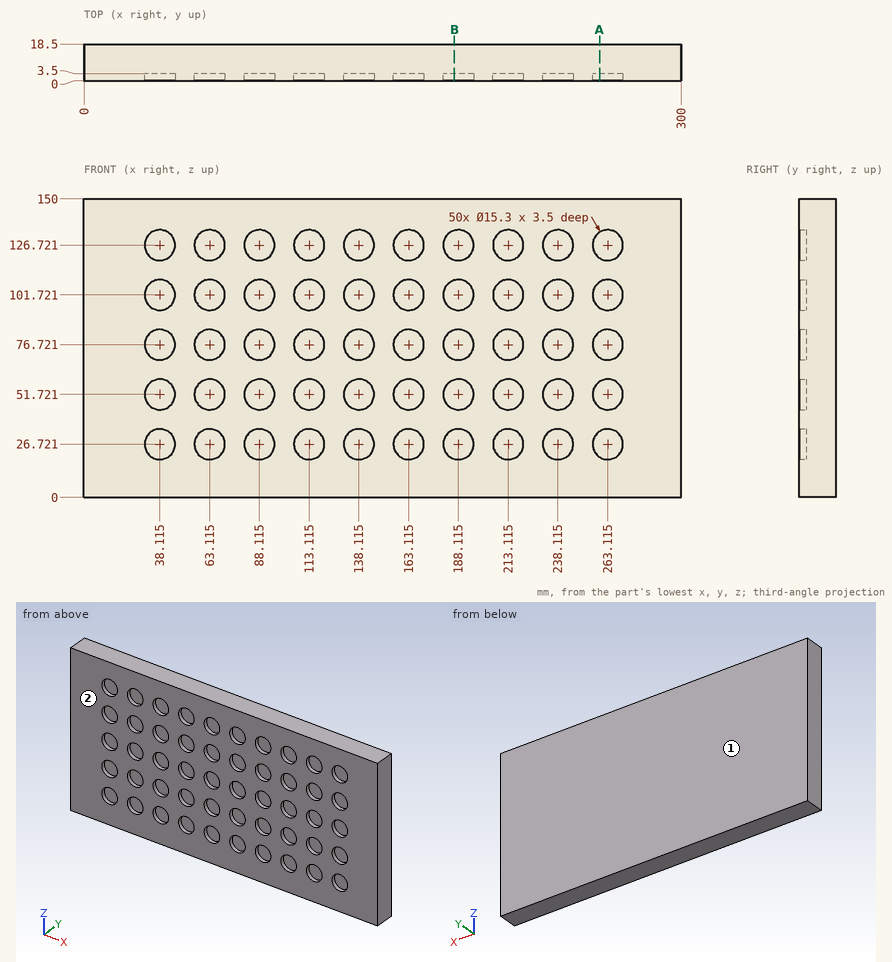
Can you work these out from the drawing? Everything is in mm from the part's minimum corner. Round coordinates to 2 decimals unless told otherwise and drop trailing zeros. Order: outer loops, then holes, each group sorted by start corner. A loop starts at its lowest first (then second) coordinate and runs counter-clockwise, first axis right, second up. Notation, with made-up numbers: M 0,43 L 58,43 A15 ccw 58,61 Z; hole C 67.25,-2.5 d9. An arc over 180 degrees is marked long. One line per question, with ' | ' between items.
1) For pin 1 Ø4.5 at (x, z) = (88, 49.5) entering from -Y, with a flat end and sliding along its axis, tell me the tip position at first contact or that it passes through.
Working result:
pin 1: y = 3.5
2) I want a section at A-A, the plane x = 259. Write out the boundary of the cut face in (y, z), then the cut area to 3 significant figures.
Working result:
outline: M 0,0 L 18.5,0 L 18.5,150 L 0,150 L 0,133.17 L 3.5,133.17 L 3.5,120.27 L 0,120.27 L 0,108.17 L 3.5,108.17 L 3.5,95.27 L 0,95.27 L 0,83.17 L 3.5,83.17 L 3.5,70.27 L 0,70.27 L 0,58.17 L 3.5,58.17 L 3.5,45.27 L 0,45.27 L 0,33.17 L 3.5,33.17 L 3.5,20.27 L 0,20.27 Z | area: 2,550 mm²
3) I need wall thicknesses on line 1 along Z through (x, y) = (133.5, 2.5); line 2 along Y through (x, z) = (36.5, 134). Which ranges of each line are inside material? Lowest first, please.
Working result:
line 1: 0 to 20.62, 32.82 to 45.62, 57.82 to 70.62, 82.82 to 95.62, 107.82 to 120.62, 132.82 to 150 | line 2: 3.5 to 18.5
4) If we mould it in two halves opening along Y, with no side actions, what happens to the marked faces 1 and 2? For each: +Y half, -Y half, draft (parallel to the pull), parting line (faces both ways), or undercut.
Working result:
face 1: +Y half | face 2: -Y half
5) I want a section at B-B, the plane x = 186. Write out the boundary of the cut face in (y, z).
Working result:
outline: M 0,0 L 18.5,0 L 18.5,150 L 0,150 L 0,134.07 L 3.5,134.07 L 3.5,119.37 L 0,119.37 L 0,109.07 L 3.5,109.07 L 3.5,94.37 L 0,94.37 L 0,84.07 L 3.5,84.07 L 3.5,69.37 L 0,69.37 L 0,59.07 L 3.5,59.07 L 3.5,44.37 L 0,44.37 L 0,34.07 L 3.5,34.07 L 3.5,19.37 L 0,19.37 Z
